Check sheet for the modelled part. Datum: model origin and axes. Units: mm. A direction names the side the tool comes from. Round coordinates to 2 decimals unless told otherwise and drop trailing zeros. Loops run counter-clockwise (first coordinate to the right, second up) from the corner with the lowest first, then second, coordinate; pieces in that order, holes last. Notation, with made-up numbers: (-23, 51) - (-7, 51) arc R29 cw to (-7, 73) - close; hole circle Ø3 at (18, -36.75). An arc over 180 degrees is marked (long way). Put each result on its own line as item: value.
```python
from build123d import *

# Parameters (mm, degrees)
BOSS_EXTRUDE1_DEPTH = 1.5
SKETCH2_W           = 5
SKETCH2_H           = 3
BOSS_EXTRUDE2_DEPTH = 3
SKETCH3_W           = 5
SKETCH3_H           = 3
BOSS_EXTRUDE3_DEPTH = 3
SKETCH4_W           = 3
SKETCH4_H           = 3
BOSS_EXTRUDE4_DEPTH = 3


with BuildPart() as part:
    # Sketch1 → Boss-Extrude1 (new body, symmetric)
    with BuildSketch(Plane(origin=(0, 0, 0), x_dir=(1, 0, 0), z_dir=(0, 1, 0))):
        Polygon((20, 15), (20, -15), (-20, -15), align=None)
    extrude(amount=BOSS_EXTRUDE1_DEPTH, both=True)

    # Sketch2 → Boss-Extrude2 (add)
    with BuildSketch(Plane(origin=(20, 0, 0), x_dir=(0, 0, -1), z_dir=(1, 0, 0))):
        with Locations((12.5, 0)):
            Rectangle(SKETCH2_W, SKETCH2_H)
        with Locations((2.5, 0)):
            Rectangle(SKETCH2_W, SKETCH2_H)
        with Locations((-7.5, 0)):
            Rectangle(SKETCH2_W, SKETCH2_H)
    extrude(amount=BOSS_EXTRUDE2_DEPTH)

    # Sketch3 → Boss-Extrude3 (add)
    with BuildSketch(Plane.XY.offset(15)):
        with Locations((17.5, 0)):
            Rectangle(SKETCH3_W, SKETCH3_H)
        with Locations((7.5, 0)):
            Rectangle(SKETCH3_W, SKETCH3_H)
        with Locations((-2.5, 0)):
            Rectangle(SKETCH3_W, SKETCH3_H)
        with Locations((-12.5, 0)):
            Rectangle(SKETCH3_W, SKETCH3_H)
    extrude(amount=BOSS_EXTRUDE3_DEPTH)

    # Sketch4 → Boss-Extrude4 (add)
    with BuildSketch(Plane(origin=(20, 0, 0), x_dir=(0, 0, -1), z_dir=(1, 0, 0))):
        with Locations((-16.5, 0)):
            Rectangle(SKETCH4_W, SKETCH4_H)
    extrude(amount=BOSS_EXTRUDE4_DEPTH)


solid = part.part
```
Item 1: Section check C-C on z = -12. Enter the section's corners in (x, y).
Filled sheet:
outline: (16, -1.5) - (23, -1.5) - (23, 1.5) - (16, 1.5) - close
Item 2: Go/stop test with flat-tipped pins: pin 1 (1.5 mm diameter, centred on y = -0.5, z = 1.5, fed in from +X); pin 2 (1.5 mm diameter, centred on y = 0.5, z = 17, fed in from -X); pin 3 (1.5 mm diameter, centred on x = 3.5, y = -0.5, fed in from +Z). Record where each tip stops, or that it passes through.
Filled sheet:
pin 1: x = 20
pin 2: x = -15
pin 3: z = 15
Item 3: Release check for a two-part mould opening along X. For faces 6 (the flat face through (6, -1.5, 5)), 7 (the flat face through (-7, 0, 15)), 8 (the flat face through (20, 0, -8)) record: +X half, -X half, draft (parallel to the pull), parting line (faces both ways), or undercut.
Filled sheet:
face 6: draft
face 7: undercut
face 8: +X half
Item 4: Section check B-B on x = -3. Enter the section's corners in (y, z), then the cut area to 4 significant figures.
Filled sheet:
outline: (-1.5, 2.25) - (1.5, 2.25) - (1.5, 18) - (-1.5, 18) - close
area: 47.25 mm²
Item 5: Tool access check on faces 1 (the flat face through (21, 0, -15)), 2 (the flat face through (19, 0, 18)), 3 (the flat face through (-17, 0, 15)), 4 (the flat face through (-5, 0, 16)), 5 (the flat face through (21, 0, -5)). Record the directions out of +Z, -Z, +X, -X, +Y, -Y that give a thin tool (end or side, any length) a straight path to the whole face; none if there is none.
Filled sheet:
face 1: -Z, +X, -X, +Y, -Y
face 2: +Z, +X, -X, +Y, -Y
face 3: +Z, -X, +Y, -Y
face 4: +Z, +Y, -Y
face 5: +X, +Y, -Y
Item 6: Thickness scan on line 1 (X direction, y = -0.4, z = 7.5); line 2 (X direction, y = -0.75, z = 1); line 3 (Z direction, x = 11.5, y = 1.25) (3 decimals). Record the ranges inside material, lowest first. Write a range as from..to.
Filled sheet:
line 1: -10..23
line 2: -1.33..20
line 3: -8.625..15
